The listing builds one solid part. Answer for the finished solid, in the listing's coordinates (mm). Face numbers are marked on the shaded views. A direction names the side the tool comes from. Coordinates: 2 decimals unless noted, no trailing zeros. Loops run counter-clockwise (first coordinate to the right, second up) from the corner with the lowest first, then second, coordinate; pieces in that order, holes last. Notation, with made-up numbers: (48, 86.5) - (55, 86.5) arc R21 cw to (55, 97.5) - close; hole circle Ø8 at (34.5, 63). An arc over 180 degrees is marked (long way). Return JSON: item names as keys, results as strings. Group by question number.
1. The mould has two halves that part along Z. Classify the marked faces 4, 5 and 6: pulls with the +Z half, pulls with the -Z half, needs draft (parallel to the pull), parting line crosses it, or undercut.
2. Find the intervals of material crossed by line 1 along X through (y, z) = (2, -30); line 2 along Z through (x, y) = (15, 7); line 3 along X through (y, z) = (13, -30), in increasing order.
3. Section C-C (y = -2) is taken. Write down the section's boundary in (x, z), and give its area (3 significant figures).
4. Each of these flat-tipped pins is pushed along its axis until it touches: P1, Ø24, axis at x = 74, z = -30.5, coming from the +Y side; P2, Ø1.5, axis at x = 18, z = -13.5, coming from the -Y side; P3, Ø3, axis at y = 28, z = -16.5, coming from the +X side. Where does it stop, or does it pass through?
5. Which of the six approach directions +Z, -Z, +X, -X, +Y, -Y give full straight-line access (tool end or side, diameter ignored) to the marked faces 1, 2 and 3?
6. Section A-A (z = -30) is taken. State how many separate pieces and enclosed holes the cut face has, and give its area (3 significant figures).
```python
from build123d import *

# Parameters (mm, degrees)
SKETCH1_W               = 60
SKETCH1_H               = 18
BOSS_EXTRUDE1_DEPTH     = 100
SKETCH6_R               = 7.5
CUT_EXTRUDE1_DEPTH      = 123.049170419
CUT_EXTRUDE1_DEPTH_BACK = 123.049170419
SKETCH7_R               = 4.551669689


with BuildPart() as part:
    # Sketch1 → Boss-Extrude1 (new body)
    with BuildSketch(Plane(origin=(0, 0, 0), x_dir=(0, 0, -1), z_dir=(1, 0, 0))):
        with Locations((30, 9)):
            Rectangle(SKETCH1_W, SKETCH1_H)
        Polygon((41.010615422, 0), (20.608108108, 0), (15, -4.73), (45, -4.73), align=None)
    extrude(amount=BOSS_EXTRUDE1_DEPTH)

    # Sweep5: sweep along a path in Sketch3
    with BuildLine(Plane(origin=(0, 0, 0), x_dir=(1, 0, 0), z_dir=(0, 1, 0))) as sweep5_path:
        Line((30, 0), (70, 60))
    # Sketch2 → Sweep5 (sweep)
    with BuildSketch(Plane.XY):
        with BuildLine():
            Line((7.550055679, 18), (52.449944321, 18))
            ThreePointArc((52.449944321, 18), (49.32222811, 19.099052512), (47.569521642, 21.913043478))
            ThreePointArc((47.569521642, 21.913043478), (30, 36), (12.430478358, 21.913043478))
            ThreePointArc((12.430478358, 21.913043478), (10.67777189, 19.099052512), (7.550055679, 18))
        make_face()
    sweep(path=sweep5_path.line)

    # Cut-Sweep3: sweep along a path in Sketch3<4>
    with BuildLine(Plane(origin=(0, 0, 0), x_dir=(1, 0, 0), z_dir=(0, 1, 0))) as cut_sweep3_path:
        Line((30, 0), (70, 60))
    # Sketch6 → Cut-Sweep3 (sweep, cut)
    with BuildSketch(Plane(origin=(0, 0, -60), x_dir=(-1, 0, 0), z_dir=(0, 0, -1))):
        with Locations((-69.99646769, 18)):
            Circle(SKETCH6_R)
    sweep(path=cut_sweep3_path.line, mode=Mode.SUBTRACT)

    # Sketch7 → Cut-Extrude1 (cut, two sides: drawn at the far end of the back side and taken through both)
    with BuildSketch(Plane(origin=(0, 0, 0), x_dir=(1, 0, 0), z_dir=(0, 1, 0)).offset(-CUT_EXTRUDE1_DEPTH_BACK)):
        with Locations(Location((15, 30, 0), (0, 0, 270))):
            Circle(SKETCH7_R)
        with Locations(Location((84.999992632, 30.022710288, 0), (0, 0, 270))):
            Circle(SKETCH7_R)
    extrude(amount=CUT_EXTRUDE1_DEPTH + CUT_EXTRUDE1_DEPTH_BACK, mode=Mode.SUBTRACT)


solid = part.part
```
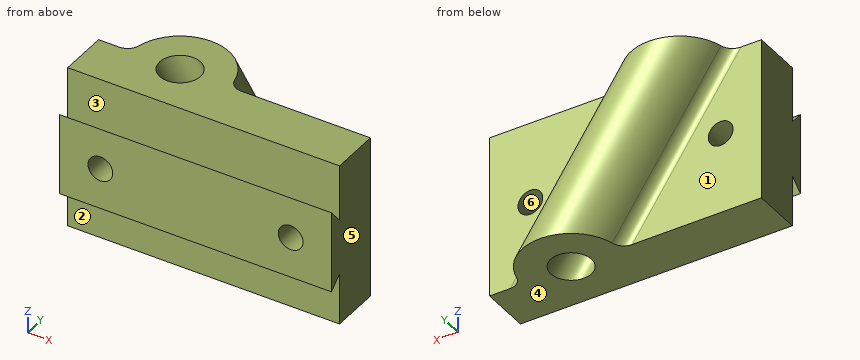
The answers:
{
 "1": {"face 4": "pulls with the -Z half", "face 5": "needs draft", "face 6": "undercut"},
 "2": {"line 1": "x = 0 to 10.45, 19.55 to 80.45, 89.55 to 100", "line 2": "z = -60 to -34.55, -25.45 to 0", "line 3": "x = 0 to 10.45, 19.55 to 44.41, 55.59 to 80.45, 89.55 to 100"},
 "3": {"outline": "(0, -42.7) - (100, -42.7) - (100, -18.24) - (0, -18.24) - close; hole circle Ø9.1 at (15, -30); hole circle Ø9.1 at (85, -30.02)", "area": "2,320 mm2"},
 "4": {"P1": "stops at y = 33.44", "P2": "stops at y = 0", "P3": "stops at x = 57.33"},
 "5": {"face 1": "-Z, -X, +Y", "face 2": "-Z, +X, -X", "face 3": "+Z, +X, -X"},
 "6": {"separate pieces": "3", "enclosed holes": "1", "area": "2,200 mm2"}
}
